```python
from build123d import *

# Parameters (mm, degrees)
BOSS_EXTRUDE1_DEPTH = 25
SKETCH2_W           = 2
SKETCH2_H           = 4
BOSS_EXTRUDE2_DEPTH = 5
SKETCH3_R           = 12
BOSS_EXTRUDE3_DEPTH = 28
SKETCH4_R           = 7
BOSS_EXTRUDE4_DEPTH = 2
SKETCH5_R           = 1
CUT_EXTRUDE1_DEPTH  = 5
BOSS_EXTRUDE5_DEPTH = 19


with BuildPart() as part:
    # Sketch1 → Boss-Extrude1 (new body)
    with BuildSketch(Plane.XY):
        with BuildLine():
            Line((7.5, -7), (7.5, 7))
            ThreePointArc((7.5, 7), (0, 10), (-7.5, 7))
            Line((-7.5, 7), (-7.5, -7))
            ThreePointArc((-7.5, -7), (0, -10), (7.5, -7))
        make_face()
    extrude(amount=BOSS_EXTRUDE1_DEPTH)

    # Sketch2 → Boss-Extrude2 (add)
    with BuildSketch(Plane(origin=(0, 0, 0), x_dir=(-1, 0, 0), z_dir=(0, 0, -1))):
        with Locations((0, 5)):
            Rectangle(SKETCH2_W, SKETCH2_H)
        with Locations((0, -5)):
            Rectangle(SKETCH2_W, SKETCH2_H)
    extrude(amount=BOSS_EXTRUDE2_DEPTH)

    # Sketch3 → Boss-Extrude3 (add)
    with BuildSketch(Plane.XY.offset(25)):
        Circle(SKETCH3_R)
    extrude(amount=BOSS_EXTRUDE3_DEPTH)

    # Sketch4 → Boss-Extrude4 (add)
    with BuildSketch(Plane.XY.offset(53)):
        Circle(SKETCH4_R)
    extrude(amount=BOSS_EXTRUDE4_DEPTH)

    # Sketch5 → Cut-Extrude1 (cut)
    with BuildSketch(Plane.XY.offset(53)):
        with Locations((-6.363961031, 6.363961031)):
            Circle(SKETCH5_R)
        with Locations((6.363961031, 6.363961031)):
            Circle(SKETCH5_R)
        with Locations((6.363961031, -6.363961031)):
            Circle(SKETCH5_R)
        with Locations((-6.363961031, -6.363961031)):
            Circle(SKETCH5_R)
    extrude(amount=-CUT_EXTRUDE1_DEPTH, mode=Mode.SUBTRACT)

    # Sketch6 → Boss-Extrude5 (add)
    with BuildSketch(Plane.XY.offset(55)):
        with BuildLine():
            Line((-1.857593316, -2.355705218), (1.857593316, -2.355705218))
            ThreePointArc((1.857593316, -2.355705218), (0, 3), (-1.857593316, -2.355705218))
        make_face()
    extrude(amount=BOSS_EXTRUDE5_DEPTH)


solid = part.part
```
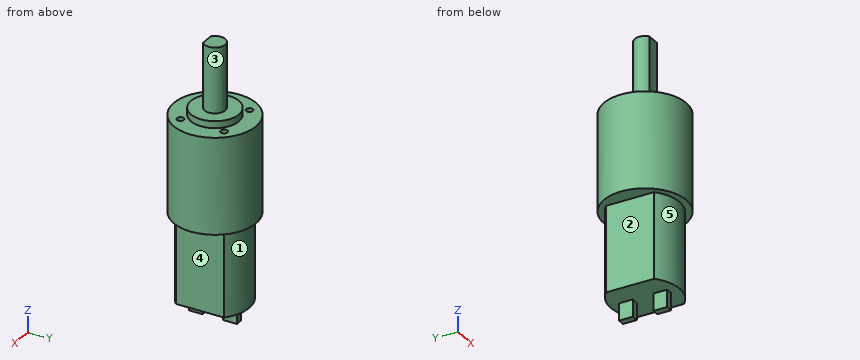
Here's how the part is built. I have some questions about the finished solid (model axes, mm). Face numbers are marked on the shaded views. A direction names the side the tool comes from. Round coordinates to 2 decimals unless told otherwise and drop trailing zeros. Order: outer loops, then holes, each group sorted by start corner. A loop starts at its lowest first (then second) coordinate and runs counter-clockwise, first axis right, second up. Notation, with made-up numbers: M -15,-33.75 L 19,-33.75 A28 cw 19,-14.75 Z; hole C 45.5,75 d5. An arc over 180 degrees is marked long. Answer in a Markdown table with one row per item.
Item 1: For the marked faces 1, 2, 3, 4 and 5, which set-ups out of +Z, -Z, +X, -X, +Y, -Y let a thin tool reach every point of the face, with its end or its side?
A:
| item | result |
|---|---|
| face 1 | -Z, +Y |
| face 2 | -Z, -X, +Y, -Y |
| face 3 | +Z |
| face 4 | -Z, +X, +Y, -Y |
| face 5 | -Z, -Y |
Item 2: Imagine slicing it at A-A, the plane y = 0. Write out the boundary of the cut face in (x, z).
A:
| item | result |
|---|---|
| outline | M -12,25 L -7.5,25 L -7.5,0 L 7.5,0 L 7.5,25 L 12,25 L 12,53 L 7,53 L 7,55 L 3,55 L 3,74 L -3,74 L -3,55 L -7,55 L -7,53 L -12,53 Z |
Item 3: Imagine slicing it at B-B, the plane x = 0. Write out the boundary of the cut face in (y, z), and give its area (3 significant figures).
A:
| item | result |
|---|---|
| outline | M -12,25 L -10,25 L -10,0 L -7,0 L -7,-5 L -3,-5 L -3,0 L 3,0 L 3,-5 L 7,-5 L 7,0 L 10,0 L 10,25 L 12,25 L 12,53 L 7,53 L 7,55 L 3,55 L 3,74 L -2.36,74 L -2.36,55 L -7,55 L -7,53 L -12,53 Z |
| area | 1,340 mm2 |
Item 4: Imagine slicing it at D-D, the plane x = -6.25. Write out the boundary of the cut face in (y, z).
A:
| item | result |
|---|---|
| outline | M -10.24,25 L -8.02,25 L -8.02,0 L 8.02,0 L 8.02,25 L 10.24,25 L 10.24,53 L 7.36,53 L 7.36,48 L 5.37,48 L 5.37,53 L 3.15,53 L 3.15,55 L -3.15,55 L -3.15,53 L -5.37,53 L -5.37,48 L -7.36,48 L -7.36,53 L -10.24,53 Z |
Item 5: I'm going to push flat-ended pins straight in: pin 1 (1.6 mm diameter, centred on x = -6.36, y = 6.36, fed in from -Z); pin 2 (2 mm diameter, centred on y = -4.5, z = -2, fed in from -X); pin 3 (3 mm diameter, centred on y = -5.5, z = -2, fed in from +X). Where does each tip first touch, or does it pass through?
A:
| item | result |
|---|---|
| pin 1 | stops at z = 0 |
| pin 2 | stops at x = -1 |
| pin 3 | stops at x = 1 |
Item 6: If I drill on L1, parallel to Z at x = -8, y = -8; L2, parallel to Z at x = 1.5, y = -4.5; L3, parallel to X at y = 4, z = 2, over which ranges is the centre line in solid material (lowest first)? Write a range as from..to.
A:
| item | result |
|---|---|
| L1 | z = 25..53 |
| L2 | z = 0..55 |
| L3 | x = -7.5..7.5 |
Item 7: Imagine slicing it at C-C, the plane z = 1. Write out the boundary of the cut face in (x, y) (3 decimals), and give its area (3 significant figures).
A:
| item | result |
|---|---|
| outline | M -7.5,-7 A10.875 ccw 7.5,-7 L 7.5,7 A10.875 ccw -7.5,7 Z |
| area | 272 mm2 |
